CAD build for the part. Positions are in the model's coordinates, mm. Face numbers are marked on the shaded views. A direction names the side the tool comes from. Coordinates: 2 decimals unless noted, no trailing zeros. Order: outer loops, then holes, each group sorted by start corner. A loop starts at its lowest first (then second) coordinate and runs counter-clockwise, first axis right, second up. Notation, with made-up numbers: (77, -21.5) - (127, -21.5) arc R13 cw to (127, -6.5) - close; hole circle Ø9 at (37.5, -31.5). An arc over 180 degrees is marked (long way). Write each question's results on one line, items separated by ' | '. Start each with the question number.
Q1. Band-saw the part on D-D, the plane z = 3.75. Write the cut outline in (x, y).
Q2. Band-saw the part on A-A, the plane z = 2. Write the cut outline in (x, y).
Q3. Pull direction X, two halves, no side cores. Call the marked faces 3, 4 and 5: released by +X, released by -X, zero draft, split by the parting line, or undercut.
Q4. Which spindle directions (+Z, -Z, +X, -X, +Y, -Y) get a long thin tool onto all of the face, cutting with end or side? Do the marked faces 1 and 2. Say none if no direction does.
Q5. Band-saw the part on B-B, the plane y = 5. Write the cut outline in (x, z), then the cut area to 3 significant figures.
Q6. Wall check: probe 1 along Y at (x, z) = (-1, -2.5); probe 2 along X at (y, z) = (6, -1.5); probe 3 along Z at (x, y) = (-0.75, 3.25). Give the ranges that are in metal, low to high.
Q7. Band-saw the part on C-C, the plane x = -5.25. Write the cut outline in (y, z).
Q8. Pin check, flat tips, straight feed: P1, Ø2, axis at x = 0, z = 0, coming from the +Y side; P2, Ø1.5, axis at x = 4, z = -0.5, coming from the -Y side; P3, Ø1, axis at x = -3, y = 2, coming from the -Z side; P4, Ø1.5, axis at x = 4.5, y = 1, coming from the +Z side. Stop position of each tip, or through.
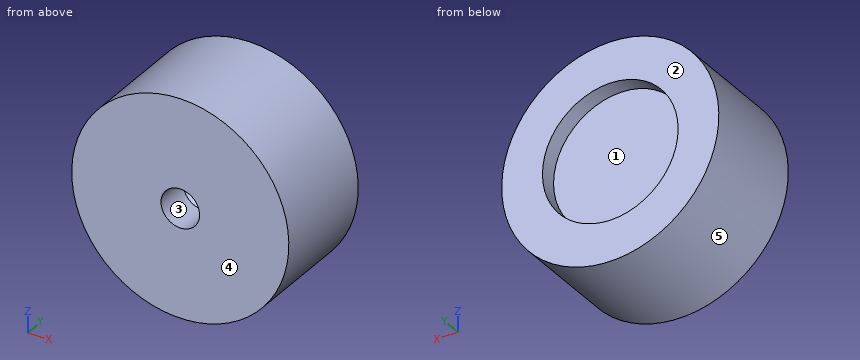
```python
from build123d import *

# Parameters (mm, degrees)
SKETCH1_R                 = 6.35
BOSS_EXTRUDE1_DEPTH       = 6.35
SKETCH2_R                 = 3.96875
CUT_EXTRUDE1_DEPTH        = 1.016
F_4_40_TAPPED_HOLE1_D     = 2.2606
F_4_40_TAPPED_HOLE1_DEPTH = 2.032
F_4_40_TAPPED_HOLE1_TIP   = 0.679152758


with BuildPart() as part:
    # Sketch1 → Boss-Extrude1 (new body)
    with BuildSketch(Plane(origin=(0, 0, 0), x_dir=(1, 0, 0), z_dir=(0, 1, 0))):
        with Locations(Location((0, 0, 0), (0, 0, 270))):
            Circle(SKETCH1_R)
    extrude(amount=BOSS_EXTRUDE1_DEPTH)

    # Sketch2 → Cut-Extrude1 (cut)
    with BuildSketch(Plane(origin=(0, 6.35, 0), x_dir=(1, 0, 0), z_dir=(0, 1, 0))):
        with Locations(Location((0, 0, 0), (0, 0, 270))):
            Circle(SKETCH2_R)
    extrude(amount=-CUT_EXTRUDE1_DEPTH, mode=Mode.SUBTRACT)

    # #4-40 Tapped Hole1
    with Locations(Plane(origin=(0, 0, 0), x_dir=(-1, 0, 0), z_dir=(0, -1, 0))):
        with Locations((0, 0)):
            Hole(F_4_40_TAPPED_HOLE1_D / 2, depth=F_4_40_TAPPED_HOLE1_DEPTH)
            with Locations((0, 0, -(F_4_40_TAPPED_HOLE1_DEPTH + F_4_40_TAPPED_HOLE1_TIP / 2))):  # 118° drill point
                Cone(0, F_4_40_TAPPED_HOLE1_D / 2, F_4_40_TAPPED_HOLE1_TIP, mode=Mode.SUBTRACT)


solid = part.part
```
Results below:
1) outline: (-5.12, 0) - (5.12, 0) - (5.12, 6.35) - (1.3, 6.35) - (1.3, 5.33) - (-1.3, 5.33) - (-1.3, 6.35) - (-5.12, 6.35) - close
2) outline: (-6.03, 0) - (6.03, 0) - (6.03, 6.35) - (3.43, 6.35) - (3.43, 5.33) - (-3.43, 5.33) - (-3.43, 6.35) - (-6.03, 6.35) - close
3) face 3: undercut | face 4: zero draft | face 5: split by the parting line
4) face 1: +Y | face 2: +Z, -Z, +X, -X, +Y
5) outline: circle Ø12.7 at (0, 0) | area: 127 mm²
6) probe 1: y = 0 to 5.33 | probe 2: x = -6.17 to -3.67, 3.67 to 6.17 | probe 3: z = -6.31 to 6.31
7) outline: (0, -3.57) - (6.35, -3.57) - (6.35, 3.57) - (0, 3.57) - close
8) P1: stops at y = 5.33 | P2: stops at y = 0 | P3: stops at z = -5.84 | P4: stops at z = 5.12
